The drawing under review shows one solid part. Ordinate dimensions are in mm from its lowest x, y, z. Round coordinates to 2 decimals unless told otherwise and drop trailing zeros. Write each loop counter-clockwise with the first axis right and the second up, starting at its lowest first coordinate (ties: lowest second). Pieces come first, ordered by that corner, then holes. Notation, with made-up numbers: M -11,16 L 26,16 A22 ccw 26,34 Z; hole C -30.5,50.5 d9. An arc over 180 degrees is marked long. Write item = value, one per line. Start each with the question number.
Item 1: Take a section at B-B, the plane y = 3.75. Give the boundary of the cut face in (x, z), plus the area to 3 significant figures.
Item 2: To check wall thickness, follow line 1 along Y through (x, z) = (7.5, 1.95); line 2 along Y through (x, z) = (3.25, 1.7); line 3 along Z through (x, y) = (3.75, 6.25). State the ranges of each line that lie inside material, in increasing order.
Item 3: Take a section at A-A, the plane x = 5.25. Give the boundary of the cut face in (y, z).
Item 4: For pin 1 Ø1 at (x, y) = (6, 10) entering from -Z, flat-tipped, find the tip position at first contact; note if it passes through.
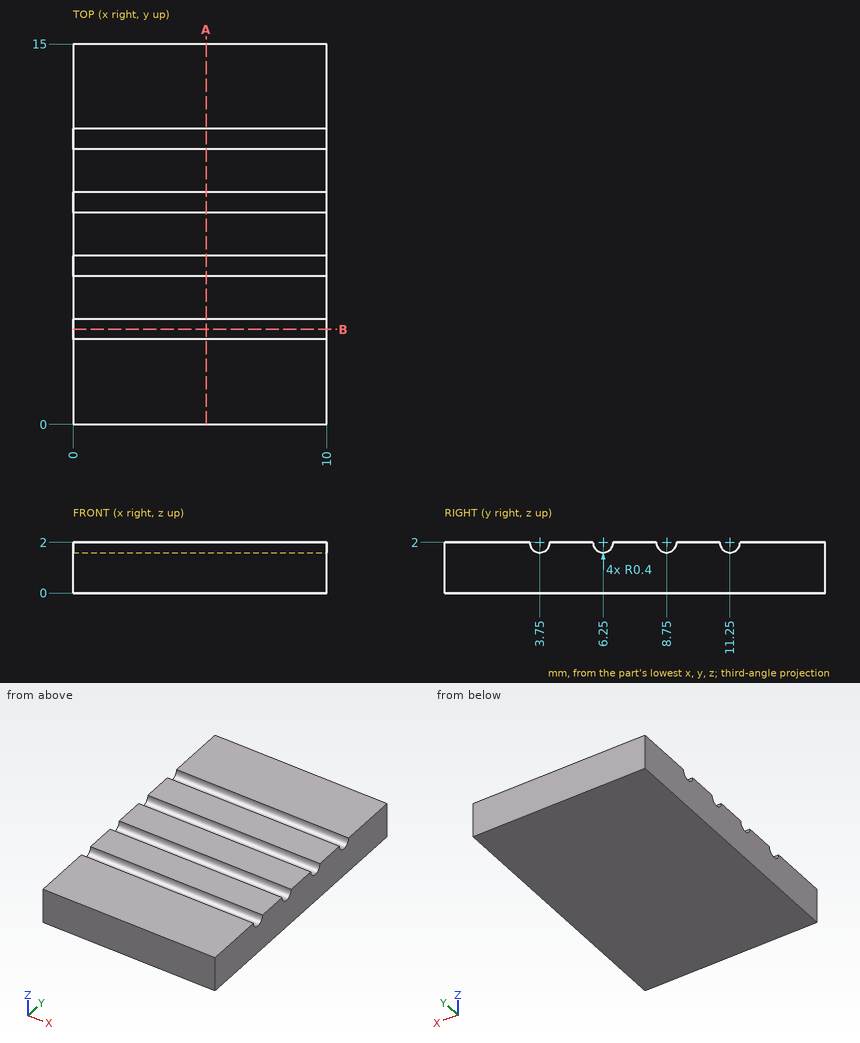
Response values:
q1.outline = M 0,0 L 10,0 L 10,1.6 L 0,1.6 Z
q1.area = 16.0 mm2
q2.line_1 = 0 to 3.35, 4.15 to 5.85, 6.65 to 8.35, 9.15 to 10.85, 11.65 to 15
q2.line_2 = 0 to 3.49, 4.01 to 5.99, 6.51 to 8.49, 9.01 to 10.99, 11.51 to 15
q2.line_3 = 0 to 1.6
q3.outline = M 0,0 L 15,0 L 15,2 L 11.65,2 A0.4 cw 10.85,2 L 9.15,2 A0.4 cw 8.35,2 L 6.65,2 A0.4 cw 5.85,2 L 4.15,2 A0.4 cw 3.35,2 L 0,2 Z
q4.pin_1 = 0
